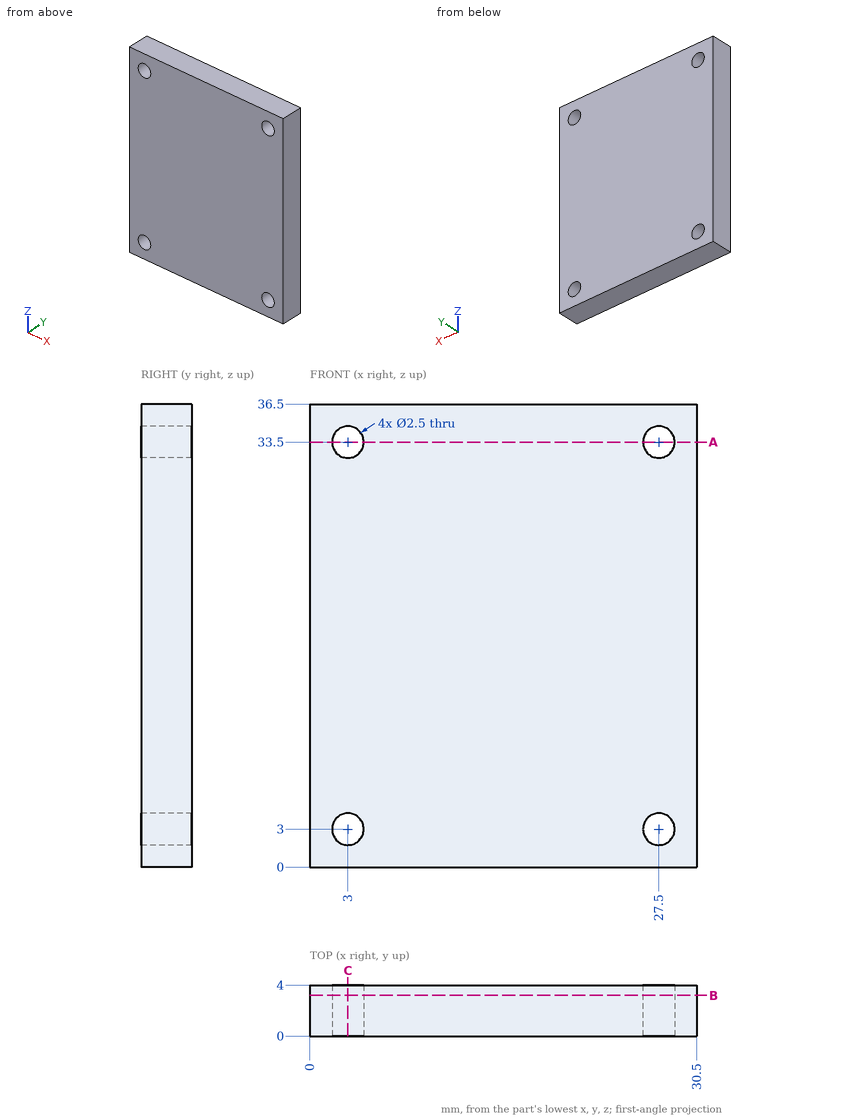
Here's the drawing with two shaded views (mm, measured from the low corner). I have some questions. Give positions to 0.01 mm unless a question says otherwise; leave off trailing zeros. Order: outer loops, then holes, each group sorted by start corner. A loop starts at its lowest first (then second) coordinate and runs counter-clockwise, first axis right, second up. Notation, with made-up numbers: (-3.5, -18) -> (35.5, -18) arc R9 ccw to (35.5, -4) -> close; hole circle Ø3 at (70.5, -8). An arc over 180 degrees is marked (long way). Use a Markdown table: item, result. Add a question column.
Item 1: Imagine slicing it at B-B on y = 3.2. Please give me the cut outline in (x, z), plus the area to 3 significant figures.
Item 2: I need wall thicknesses on line 1 (X direction, y = 2.7, z = 33.5); line 2 (Z direction, x = 3, y = 2.65); line 3 (Z direction, x = 3.5, y = 2.95). Which ranges of each line are inside material? Lowest first, please.
Item 3: Imagine slicing it at C-C on x = 3. Please give me the cut outline in (y, z).
Item 4: Imagine slicing it at A-A on z = 33.5. Please give me the cut outline in (x, y).
Data:
| question | item | result |
|---|---|---|
| 1 | outline | (0, 0) -> (30.5, 0) -> (30.5, 36.5) -> (0, 36.5) -> close; hole circle Ø2.5 at (3, 3); hole circle Ø2.5 at (3, 33.5); hole circle Ø2.5 at (27.5, 3); hole circle Ø2.5 at (27.5, 33.5) |
| 1 | area | 1,090 mm² |
| 2 | line 1 | x = 0 to 1.75, 4.25 to 26.25, 28.75 to 30.5 |
| 2 | line 2 | z = 0 to 1.75, 4.25 to 32.25, 34.75 to 36.5 |
| 2 | line 3 | z = 0 to 1.85, 4.15 to 32.35, 34.65 to 36.5 |
| 3 | outline | (0, 0) -> (4, 0) -> (4, 1.75) -> (0, 1.75) -> close; (0, 4.25) -> (4, 4.25) -> (4, 32.25) -> (0, 32.25) -> close; (0, 34.75) -> (4, 34.75) -> (4, 36.5) -> (0, 36.5) -> close |
| 4 | outline | (0, 0) -> (1.75, 0) -> (1.75, 4) -> (0, 4) -> close; (4.25, 0) -> (26.25, 0) -> (26.25, 4) -> (4.25, 4) -> close; (28.75, 0) -> (30.5, 0) -> (30.5, 4) -> (28.75, 4) -> close |
